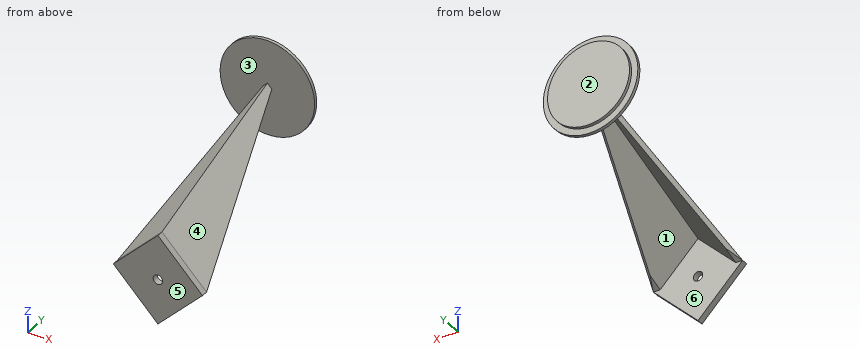
from build123d import *

# Parameters (mm, degrees)
SKETCH1_R           = 1.5
BOSS_EXTRUDE2_DEPTH = 2
BOSS_EXTRUDE3_DEPTH = 55
CUT_EXTRUDE1_DEPTH  = 2
CUT_EXTRUDE2_DEPTH  = 2
SKETCH8_R           = 15
BOSS_EXTRUDE6_DEPTH = 2
CUT_EXTRUDE3_START  = -1
SKETCH12_R          = 15
SKETCH12_R_2        = 13
CUT_EXTRUDE3_DEPTH  = 1


with BuildPart() as part:
    # Sketch1 → Boss-Extrude2 (new body)
    with BuildSketch(Plane(origin=(0, 0, 0), x_dir=(1, 0, 0), z_dir=(0, 1, 0))):
        Polygon((0, 14.142135624), (-14.142135624, 0), (0, -14.142135624), (14.142135624, 0), align=None)
        with Locations(Location((0, 0, 0), (0, 0, 270))):
            Circle(SKETCH1_R, mode=Mode.SUBTRACT)
    extrude(amount=BOSS_EXTRUDE2_DEPTH)

    # Sketch3 → Boss-Extrude3 (add, along a direction that is not the sketch's normal)
    with BuildSketch(Plane(origin=(0, 2, 0), x_dir=(1, 0, 0), z_dir=(0, 1, 0))):
        Polygon((0, -14.142135624), (14.142135624, 0), (12, 0), (0, -12), (-12, 0), (-14.142135624, 0), align=None)
    extrude(amount=BOSS_EXTRUDE3_DEPTH, dir=(0, 0.9396926207859093, 0.34202014332566616))

    # Sketch5 → Cut-Extrude1 (cut)
    with BuildSketch(Plane(origin=(6.290436868, -2.289531781, 6.290436868), x_dir=(0.643493123501823, -0.23421234290964707, -0.7287394448186825), z_dir=(0.6847910787717363, -0.24924356936395234, 0.6847910787717364))):
        Polygon((8.63194234, 6.716280495), (-17.181272543, 55.28250268), (-34.646941723, 50.929296953), align=None)
    extrude(amount=-CUT_EXTRUDE1_DEPTH, mode=Mode.SUBTRACT)

    # Sketch6 → Cut-Extrude2 (cut)
    with BuildSketch(Plane(origin=(-6.290436868, -2.289531781, 6.290436868), x_dir=(0.6434931235018196, 0.23421234290964207, 0.7287394448186869), z_dir=(-0.6847910787717418, -0.24924356936395037, 0.6847910787717316))):
        Polygon((17.181272543, 55.28250268), (34.646941723, 50.929296953), (-8.63194234, 6.716280495), align=None)
    extrude(amount=-CUT_EXTRUDE2_DEPTH, mode=Mode.SUBTRACT)

    # Sketch8 → Boss-Extrude6 (add)
    with BuildSketch(Plane(origin=(0, 53.683094143, 0), x_dir=(1, 0, 0), z_dir=(0, 1, 0))):
        with Locations(Location((0, -31.539029944, 0), (0, 0, 270))):
            Circle(SKETCH8_R)
    extrude(amount=BOSS_EXTRUDE6_DEPTH)

    # Sketch12 → Cut-Extrude3 (cut)
    with BuildSketch(Plane(origin=(0, 55.683094143, 0), x_dir=(1, 0, 0), z_dir=(0, 1, 0)).offset(CUT_EXTRUDE3_START)):
        with Locations(Location((0, -31.539029944, 0), (0, 0, 270))):
            Circle(SKETCH12_R)
        with Locations(Location((0, -31.539029944, 0), (0, 0, 270))):
            Circle(SKETCH12_R_2, mode=Mode.SUBTRACT)
    extrude(amount=CUT_EXTRUDE3_DEPTH, mode=Mode.SUBTRACT)


solid = part.part
Can you work these out from the model? Positions are in its coordinate system, mm. Face numbers are marked on the shaded views. A direction names the side the tool comes from. Coordinates: 2 decimals unless noted, no trailing zeros. Write each loop counter-clockwise with the first axis right and the second up, starting at its lowest first coordinate (ties: lowest second). Pieces come first, ordered by that corner, then holes. Notation, with made-up numbers: (81.5, 32.25) -> (118.5, 32.25) arc R23 cw to (118.5, 58.25) -> close; hole circle Ø10 at (36, -14.5). An arc over 180 degrees is marked (long way). Answer as CSV lines item,"result".
1) If I drill on line 1 (X direction, y = 0.7, z = 0); line 2 (Y direction, x = -7.5, z = -6); line 3 (X direction, y = 17.5, z = 9), over which ranges is the centre line in solid material (lowest first)? Write a range as from..to.
Check result:
line 1,"-14.14..-1.5, 1.5..14.14"
line 2,"0..2"
line 3,"-9.98..-8.64, 8.64..9.98"
2) If we section it at D-D on z = 9.5: Please give me the cut outline in (x, y).
Check result:
outline,"(-10.31, 17.57) -> (-4.64, 2) -> (-4.64, 0) -> (4.64, 0) -> (4.64, 2) -> (10.31, 17.57) -> (8.9, 19.58) -> (2.5, 2) -> (-2.5, 2) -> (-8.9, 19.58) -> close"
3) If we section it at A-A on z = 23: Please give me the cut outline in (x, y), then the cut area to 3 significant figures.
Check result:
outline,"(-12.33, 53.68) -> (12.33, 53.68) -> (12.33, 54.68) -> (9.8, 54.68) -> (9.8, 55.68) -> (-9.8, 55.68) -> (-9.8, 54.68) -> (-12.33, 54.68) -> close; (-4.86, 39.69) -> (0, 26.34) -> (4.86, 39.69) -> (3.45, 41.7) -> (0, 32.22) -> (-3.45, 41.7) -> close"
area,"93.2 mm²"
4) If we section it at B-B on x = 11.25: Please give me the cut outline in (y, z).
Check result:
outline,"(0, -2.89) -> (2, -2.89) -> (2, 0.75) -> (10.03, 3.67) -> (13.74, 7.17) -> (2, 2.89) -> (0, 2.89) -> close; (53.68, 21.62) -> (54.68, 21.62) -> (54.68, 25.02) -> (55.68, 25.02) -> (55.68, 38.05) -> (54.68, 38.05) -> (54.68, 41.46) -> (53.68, 41.46) -> close"
5) If we mould it in two halves opening along Y, with no side actions, what happens to the marked faces 1, 2, 3 and 4? For each: +Y half, -Y half, draft (parallel to the pull), parting line (faces both ways), or undercut.
Check result:
face 1,"undercut"
face 2,"+Y half"
face 3,"undercut"
face 4,"-Y half"
6) Will these pins go through, and if not, where does the flat tip stop? P1, Ø12, axis at y = 7.5, z = 28, coming from the -X side; P2, Ø12, axis at x = 5.5, z = 16.5, coming from the -Y side; P3, Ø5, axis at x = 0, z = 0, coming from the +Y side; P4, Ø3, axis at x = -2, y = 49.5, coming from the -Z side.
Check result:
P1,"through"
P2,"y = 0"
P3,"y = 2"
P4,"z = 26.85"
7) On a 3-axis mill with a long thin cutter (end or side, diameter ignored), from which of +Z, -Z, +X, -X, +Y, -Y can I reach the whole of each face in a straight line? I mean the marked faces 5 and 6. Say none if no direction works.
Check result:
face 5,"+Z, -Z, +X, -X, -Y"
face 6,"-Z, +Y"
8) If we section it at C-C on y = 40.5: Please give me the cut outline in (x, z).
Check result:
outline,"(-4.66, 23.49) -> (-3.75, 22.27) -> (0, 26.01) -> (3.75, 22.27) -> (4.66, 23.49) -> (0, 28.15) -> close"
